The figure shows three views and two pictorial views of one solid part (mm, origin at its lowest corner). Answer the questions. A direction names the side the tool comes from. Give positions to 0.01 mm unless a question says otherwise; leave off trailing zeros. Order: outer loops, then holes, each group sorted by start corner. A loop starts at its lowest first (then second) coordinate and runs counter-clockwise, first axis right, second up. Notation, with made-up numbers: (78.25, 66) - (108.25, 66) arc R5 cw to (108.25, 72) - close; hole circle Ø8 at (57.5, 67.5). An arc over 180 degrees is marked (long way). Use a Markdown table: item, result. Add a question column.
1. A cutting plane is placed at A-A on x = 8. Determine the outline of the cut face in (y, z), and give its area (3 significant figures).
2. A cutting plane is placed at B-B on y = 7. Determine the outline of the cut face in (x, z).
3. A cutting plane is placed at D-D on z = 18. Determine the outline of the cut face in (x, y), and give its area (3 significant figures).
4. A cutting plane is placed at C-C on x = 16. Determine the outline of the cut face in (y, z).
5. Consider L1, parallel to X at y = 6.5, z = 6.25; L2, parallel to Y at x = 30.8, z = 4; L3, parallel to X at y = 1.5, z = 11. Determine where each line is inside the solid, lowest interval first.
6. Flat-ended cylindrical pins translate along their axes: P1, Ø12, axis at x = 16, z = 11, coming from the -Y side; P2, Ø4, axis at x = 16, z = 3, coming from the +Y side. Find the tip coordinate at first contact, or state that the pin passes through.
7. Which of the six approach directions +Z, -Z, +X, -X, +Y, -Y give full straight-line access (tool end or side, diameter ignored) to the marked faces 4 and 5?
8. For a pull along Z with two mould halves and no side action, classify the marked faces 1, 2 and 3 as released by +Z, released by -Z, zero draft, split by the parting line, or undercut.
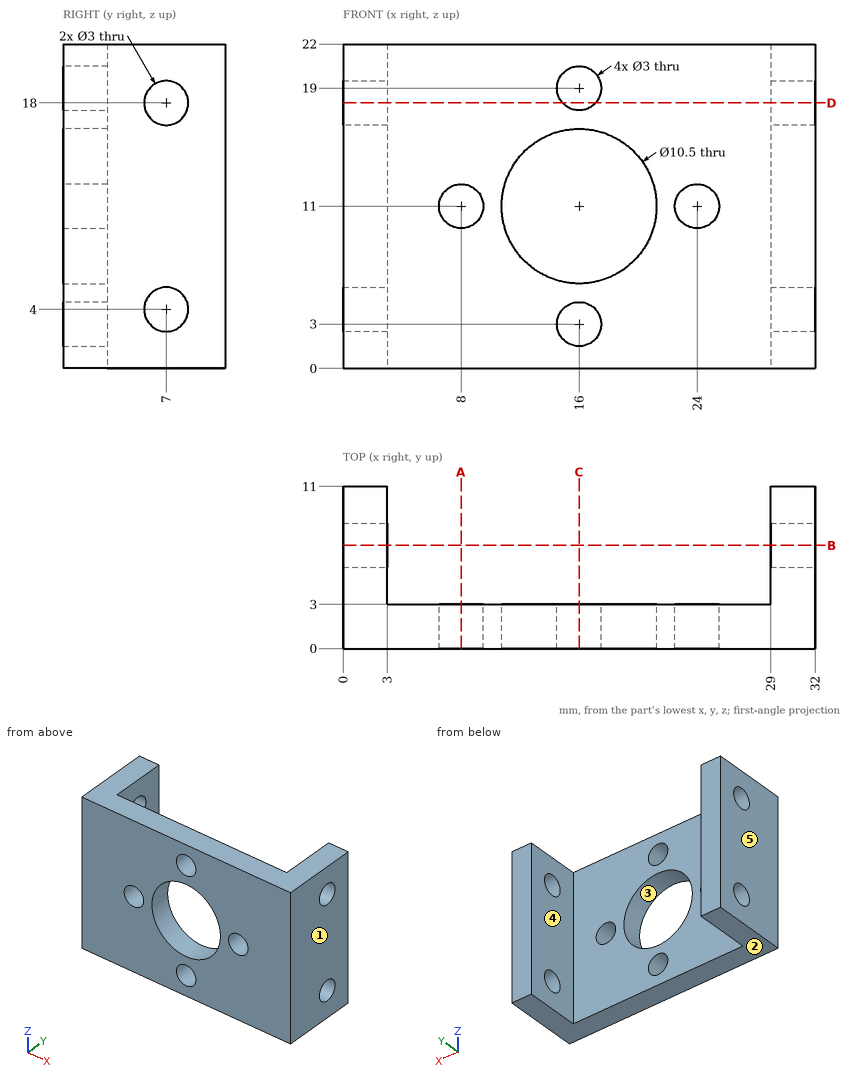
Output values:
| question | item | result |
|---|---|---|
| 1 | outline | (0, 0) - (3, 0) - (3, 9.5) - (0, 9.5) - close; (0, 12.5) - (3, 12.5) - (3, 22) - (0, 22) - close |
| 1 | area | 57.0 mm² |
| 2 | outline | (0, 0) - (3, 0) - (3, 2.5) - (0, 2.5) - close; (0, 5.5) - (3, 5.5) - (3, 16.5) - (0, 16.5) - close; (0, 19.5) - (3, 19.5) - (3, 22) - (0, 22) - close; (29, 0) - (32, 0) - (32, 2.5) - (29, 2.5) - close; (29, 5.5) - (32, 5.5) - (32, 16.5) - (29, 16.5) - close; (29, 19.5) - (32, 19.5) - (32, 22) - (29, 22) - close |
| 3 | outline | (0, 0) - (14.88, 0) - (14.88, 3) - (3, 3) - (3, 5.5) - (0, 5.5) - close; (0, 8.5) - (3, 8.5) - (3, 11) - (0, 11) - close; (17.12, 0) - (32, 0) - (32, 5.5) - (29, 5.5) - (29, 3) - (17.12, 3) - close; (29, 8.5) - (32, 8.5) - (32, 11) - (29, 11) - close |
| 3 | area | 119 mm² |
| 4 | outline | (0, 0) - (3, 0) - (3, 1.5) - (0, 1.5) - close; (0, 4.5) - (3, 4.5) - (3, 5.75) - (0, 5.75) - close; (0, 16.25) - (3, 16.25) - (3, 17.5) - (0, 17.5) - close; (0, 20.5) - (3, 20.5) - (3, 22) - (0, 22) - close |
| 5 | L1 | 0 to 3, 29 to 32 |
| 5 | L2 | 0 to 5.5, 8.5 to 11 |
| 5 | L3 | 0 to 6.5, 9.5 to 10.75, 21.25 to 22.5, 25.5 to 32 |
| 6 | P1 | y = 0 |
| 6 | P2 | y = 3 |
| 7 | face 4 | +Z, -Z, +Y |
| 7 | face 5 | +Z, -Z, -X, +Y, -Y |
| 8 | face 1 | zero draft |
| 8 | face 2 | released by -Z |
| 8 | face 3 | undercut |
